Here's how the part is built. I have some questions about the finished solid (model axes, mm). Coordinates: 2 decimals unless noted, no trailing zeros. Loops run counter-clockwise (first coordinate to the right, second up) from the corner with the lowest first, then second, coordinate; pieces in that order, holes last. Notation, with made-up numbers: (71, 43) -> (118, 43) arc R23 cw to (118, 69) -> close; hole circle Ø9 at (-29.5, 43). An arc over 180 degrees is marked (long way). Answer as a JSON object with one key per item and string values. Group by question number.
1) I want a section at D-D (y = 4.5). Write out the boundary of the cut face in (x, z), then the cut area to 3 significant figures.
2) I'm going to push a flat-ended pin straight in: pin 1 (6 mm diameter, centred on y = 4, z = 5.5, fed in from +X). Where does the tip first touch, or does it pass through?
3) I want a section at B-B (x = 0). Write out the boundary of the cut face in (y, z).
4) I want a section at C-C (y = 0). Write out the boundary of the cut face in (x, z).
5) If we mould it in two halves opening along Y, with no side actions, what happens to faces 1 (the flat face through (12, -7, 0)), 2 (the cylindrical face through (13.318, 0.751, -2.385)), 3 (the flat face through (12, 7, 0))? For each: +Y half, -Y half, draft (parallel to the pull), parting line (faces both ways), or undercut.
6) I need wall thicknesses on probe 1 along Y at (x, z) = (-12.45, 0); probe 2 along X at (y, z) = (2.75, -5); probe 3 along Z at (x, y) = (2, 3.75). Which ranges of each line are inside material? Lowest first, please. Write a range as [from, to].
7) I want a section at A-A (z = 0). Write out the boundary of the cut face in (x, y).
```python
from build123d import *

# Parameters (mm, degrees)
SKETCH1_R               = 16
SKETCH1_R_2             = 11
BOSS_EXTRUDE1_DEPTH     = 7
CUT_EXTRUDE1_DEPTH      = 24.685438565
CUT_EXTRUDE1_DEPTH_BACK = 24.685438565
SKETCH2_R               = 2.5
FILLET1_R               = 0.5


with BuildPart() as part:
    # Sketch1 → Boss-Extrude1 (new, symmetric)
    with BuildSketch(Plane(origin=(0, 0, 0), x_dir=(1, 0, 0), z_dir=(0, 1, 0))):
        with Locations(Location((0, 0, 0), (0, 0, 270))):
            Circle(SKETCH1_R)
        with Locations(Location((0, 0, 0), (0, 0, 270))):
            Circle(SKETCH1_R_2, mode=Mode.SUBTRACT)
    extrude(amount=BOSS_EXTRUDE1_DEPTH, both=True)

    # Sketch2 → Cut-Extrude1 (cut, two sides: drawn at the far end of the back side and taken through both)
    with BuildSketch(Plane(origin=(0, 0, 0), x_dir=(0, 0, -1), z_dir=(1, 0, 0)).offset(-CUT_EXTRUDE1_DEPTH_BACK)):
        Circle(SKETCH2_R)
    extrude(amount=CUT_EXTRUDE1_DEPTH + CUT_EXTRUDE1_DEPTH_BACK, mode=Mode.SUBTRACT)

    # Fillet1
    fillet1_edges = [part.edges().sort_by_distance(p)[0] for p in [
        (0, -7, -16),
        (0, 7, -16),
        (0, -7, -11),
        (0, 7, -11),
    ]]
    fillet(fillet1_edges, radius=FILLET1_R)


solid = part.part
```
Determined:
{
 "1": {"outline": "circle Ø32 at (0, 0); hole circle Ø22 at (0, 0)", "area": "424 mm^2"},
 "2": {"pin 1": "x = 15.8"},
 "3": {"outline": "(-7, -15.5) arc R0.5 ccw to (-6.5, -16) -> (6.5, -16) arc R0.5 ccw to (7, -15.5) -> (7, -11.5) arc R0.5 ccw to (6.5, -11) -> (-6.5, -11) arc R0.5 ccw to (-7, -11.5) -> close; (-7, 11.5) arc R0.5 ccw to (-6.5, 11) -> (6.5, 11) arc R0.5 ccw to (7, 11.5) -> (7, 15.5) arc R0.5 ccw to (6.5, 16) -> (-6.5, 16) arc R0.5 ccw to (-7, 15.5) -> close"},
 "4": {"outline": "(-15.8, -2.5) arc R16 ccw to (15.8, -2.5) -> (10.71, -2.5) arc R11 cw to (-10.71, -2.5) -> close; (-15.8, 2.5) -> (-10.71, 2.5) arc R11 cw to (10.71, 2.5) -> (15.8, 2.5) arc R16 ccw to start"},
 "5": {"face 1": "-Y half", "face 2": "undercut", "face 3": "+Y half"},
 "6": {"probe 1": "[-7, -2.5], [2.5, 7]", "probe 2": "[-15.2, -9.8], [9.8, 15.2]", "probe 3": "[-15.87, -10.82], [10.82, 15.87]"},
 "7": {"outline": "(-16, -6.5) arc R0.5 ccw to (-15.5, -7) -> (-11.5, -7) arc R0.5 ccw to (-11, -6.5) -> (-11, -2.5) -> (-16, -2.5) -> close; (-16, 2.5) -> (-11, 2.5) -> (-11, 6.5) arc R0.5 ccw to (-11.5, 7) -> (-15.5, 7) arc R0.5 ccw to (-16, 6.5) -> close; (11, -6.5) arc R0.5 ccw to (11.5, -7) -> (15.5, -7) arc R0.5 ccw to (16, -6.5) -> (16, -2.5) -> (11, -2.5) -> close; (11, 2.5) -> (16, 2.5) -> (16, 6.5) arc R0.5 ccw to (15.5, 7) -> (11.5, 7) arc R0.5 ccw to (11, 6.5) -> close"}
}
